The listing builds one solid part. Answer for the finished solid, in the listing's coordinates (mm). Face numbers are marked on the shaded views. A direction names the side the tool comes from. Round coordinates to 2 decimals unless told otherwise and drop trailing zeros. Loops run counter-clockwise (first coordinate to the right, second up) from the corner with the lowest first, then second, coordinate; pieces in that order, holes last. Notation, with made-up numbers: (63, 45.5) -> (74, 45.5) arc R21 ccw to (74, 57.5) -> close; hole circle Ø7 at (8.25, 72). An arc over 180 degrees is marked (long way). One line per question, with ' | ' between items.
from build123d import *

# Parameters (mm, degrees)
F0_W     = 50
F0_H     = 50
F0_R     = 3
F1_DEPTH = 5
F2_DEPTH = 5
F3_R     = 2.5
F4_DEPTH = 10


with BuildPart() as f1:
    # F0 (on Top) → F1 (new body, symmetric)
    with BuildSketch(Plane.XY):
        with Locations((25, -25)):
            Rectangle(F0_W, F0_H)
        with Locations((5, -45)):
            Circle(F0_R, mode=Mode.SUBTRACT)
        Polygon((14.2875, -30.020106), (38.09502, -30.020106), (42.85752, -30.020106), (42.85752, -34.782606), (38.09502, -34.782606), (9.525, -34.782606), (9.525, -28.575), (9.525, -19.05), (14.2875, -19.05), (14.2875, -14.2875), (9.525, -14.2875), (9.525, -9.525), (19.05, -9.525), (19.05, -19.05), (23.8125, -19.05), (23.8125, -9.525), (28.575, -9.525), (38.80062, -9.525), (44.80062, -9.525), (44.80062, -19.461621), (40.03812, -19.461621), (40.03812, -14.699121), (30.854725, -14.699121), (30.854725, -19.461621), (30.854725, -23.8125), (23.8125, -23.8125), (23.8125, -28.575), (19.05, -28.575), (19.05, -23.8125), (14.2875, -23.8125), (14.2875, -28.575), align=None, mode=Mode.SUBTRACT)
        with Locations((45, -5)):
            Circle(F0_R, mode=Mode.SUBTRACT)
    extrude(amount=F1_DEPTH, both=True)

    # F0 (on Top) → F2 (join)
    with BuildSketch(Plane.XY):
        Polygon((38.09502, -34.782606), (38.09502, -30.020106), (14.2875, -30.020106), (14.2875, -28.575), (14.2875, -23.8125), (19.05, -23.8125), (19.05, -28.575), (23.8125, -28.575), (23.8125, -23.8125), (30.854725, -23.8125), (30.854725, -19.461621), (30.854725, -14.699121), (40.03812, -14.699121), (40.03812, -19.461621), (44.80062, -19.461621), (44.80062, -9.525), (38.80062, -9.525), (28.575, -9.525), (23.8125, -9.525), (23.8125, -19.05), (19.05, -19.05), (19.05, -9.525), (9.525, -9.525), (9.525, -14.2875), (14.2875, -14.2875), (14.2875, -19.05), (9.525, -19.05), (9.525, -28.575), (9.525, -34.782606), align=None)
    extrude(amount=-F2_DEPTH)

    # F3 (on face) → F4 (join)
    with BuildSketch(Plane.XY.offset(5)):
        with Locations((5, -5)):
            Circle(F3_R)
        with Locations((45, -45)):
            Circle(F3_R)
    extrude(amount=F4_DEPTH)


solid = f1.part
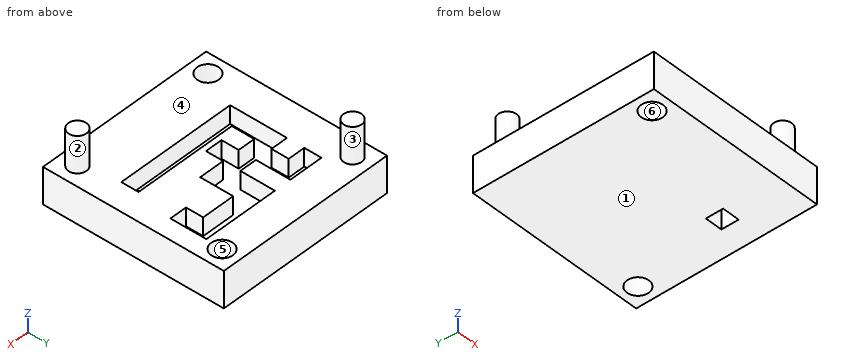
Q1. Find the intervals of material crossed by line 1 (Y direction, x = 29, z = 3.5) (1 decimal); line 2 (Y direction, x = 5, z = -1.75); line 3 (X direction, y = -21, z = 4.25) (3 decimals), in increasing order. Write a range as from..to.
Numbers:
line 1: -50..-34.8, -30..-23.8, -9.5..0 | line 2: -50..-48, -42..0 | line 3: 0..9.525, 30.855..50
Q2. Given pin 1 Ø12.5 at (x, y) = (33.5, -17) entering from +Z; pin 2 Ø5.5 at (x, y) = (5, -45) entering from -Z, each flat-ended and moving along its own axis, determine where each tip first touches the part or whether it passes through.
Numbers:
pin 1: z = 5 | pin 2: through
Q3. A cutting plane is placed at A-A on x = 5. Give the vertices of the cut face in (y, z), plus the area to 3 significant figures.
Numbers:
outline: (-50, -5) -> (-48, -5) -> (-48, 5) -> (-50, 5) -> close; (-42, -5) -> (0, -5) -> (0, 5) -> (-2.5, 5) -> (-2.5, 15) -> (-7.5, 15) -> (-7.5, 5) -> (-42, 5) -> close | area: 490 mm^2
Q4. A cutting plane is placed at C-C on z = 4. Give the number of separate pieces and of enclosed holes in the cut face, plus the area to 3 significant figures.
Numbers:
separate pieces: 1 | enclosed holes: 3 | area: 1,900 mm^2
Q5. For the marked faces 1 and 2, determine the directions among +Z, -Z, +X, -X, +Y, -Y from which every point of the face is accessible in a straight line to the end or side of a thin tool.
Numbers:
face 1: -Z, +X, -X, +Y, -Y | face 2: +Z
Q6. For a pull along Y with two mould halves and no side action, classify the marked faces 3, 4, 5 and 6 as pulls with the +Y half, pulls with the -Y half, needs draft (parallel to the pull), parting line crosses it, or undercut.
Numbers:
face 3: parting line crosses it | face 4: needs draft | face 5: undercut | face 6: undercut
Q7. A cutting plane is placed at D-D on y = -17. Give the vertices of the cut face in (x, z), plus the area to 3 significant figures.
Numbers:
outline: (0, -5) -> (50, -5) -> (50, 5) -> (44.8, 5) -> (44.8, 0) -> (40.04, 0) -> (40.04, 5) -> (30.85, 5) -> (30.85, 0) -> (23.81, 0) -> (23.81, 5) -> (19.05, 5) -> (19.05, 0) -> (14.29, 0) -> (14.29, 5) -> (0, 5) -> close | area: 417 mm^2
Q8. A cutting plane is placed at B-B on y = -5. Give the vertices of the cut face in (x, z).
Numbers:
outline: (0, -5) -> (42, -5) -> (42, 5) -> (7.5, 5) -> (7.5, 15) -> (2.5, 15) -> (2.5, 5) -> (0, 5) -> close; (48, -5) -> (50, -5) -> (50, 5) -> (48, 5) -> close
